Geometry: final body of the model. Coordinates: model frame, mm. A direction names the side the tool comes from. Give positions to 0.01 mm unless a question says otherwise; leave off trailing zeros. Loops run counter-clockwise (first coordinate to the right, second up) from the corner with the lowest first, then second, coordinate; pieces in that order, holes last. Notation, with made-up numbers: (67, 73.5) -> (95, 73.5) arc R15 ccw to (95, 90.5) -> close; hole circle Ø1 at (84, -8). An arc over 180 degrees is marked (long way). Answer in a Markdown table with one row per item. Add a question column.
1) Section query A-A (y = 148). Return the cut outline in (x, z), plus the area to 3 significant figures.
2) Line query: line 1 (Y direction, x = 0, z = 0.55); line 2 (Y direction, x = 48.5, z = 1.8); line 3 (Y direction, x = -71, z = 1.4). Output: solid intervals per line, ascending. Write a range as from..to.
3) Access query for faces 5 (the flat face through (73.772, 0.454, 0.986)), 6 (the flat face through (-61.02, 229.27, 0.99)), 7 (the flat face through (61.023, -14.957, 0.986)). Directions: +Z, -Z, +X, -X, +Y, -Y. A direction counts if a zero-diameter tool reaches every point of the face in a straight line with its end or side. Return the directions, or none.
4) Section query B-B (z = 1.3). Give the number of separate pieces and of enclosed holes in the cut face, plus the area to 3 significant figures.
5) First-contact query: P1, Ø1.3, axis at x = 74.81, y = 99.66, coming from the -Z side; P2, Ø1, axis at x = 80, z = 0.5, coming from the -Y side. Flat tips, straight axial feed; report the tip coordinate or a pass-through.
6) Draft query along Y for faces 1 (the flat face through (71.318, -10.358, 0.986)), 2 (the cylindrical face through (-58.96, 16.71, 0.99)), 3 (the cylindrical face through (59.714, 124.35, 0.986)), 4 (the flat face through (1, 109, 0)). Return one class per face: +Y half, -Y half, draft (parallel to the pull), parting line (faces both ways), or undercut.
7) Section query C-C (x = -30). Return the cut outline in (y, z), plus the area to 3 significant figures.
```python
from build123d import *

# Parameters (mm, degrees)
EXTRUDE_1_DEPTH     = 2
SKETCH_2_R          = 0.8
SKETCH_2_R_2        = 2
CUT_EXTRUDE_1_DEPTH = 10
SKETCH_3_R          = 1.5
SKETCH_3_R_2        = 1
CUT_EXTRUDE_2_DEPTH = 249.131112982
SKETCH_4_R          = 2
CUT_EXTRUDE_3_DEPTH = 10


with BuildPart() as part:
    # 草图1 → 凸台-拉伸1 (new body)
    with BuildSketch(Plane.XY):
        with BuildLine():
            Line((-52.894125512, 33.242924291), (-52.894125512, 73.242924291))
            ThreePointArc((-52.894125512, 73.242924291), (-59.898712726, 90.153493742), (-76.809282177, 97.158080957))
            Line((-76.809282177, 97.158080957), (-86.809282177, 97.158080957))
            Line((-86.809282177, 97.158080957), (-86.809282177, 117.158080957))
            Line((-86.809282177, 117.158080957), (-76.809282177, 117.158080957))
            ThreePointArc((-76.809282177, 117.158080957), (-59.898712726, 124.162668171), (-52.894125512, 141.073237622))
            Line((-52.894125512, 141.073237622), (-52.894125512, 181.073237622))
            ThreePointArc((-52.894125512, 181.073237622), (-58.833242973, 197.390828739), (-69.995132678, 210.693050895))
            Line((-69.995132678, 210.693050895), (-77.655577109, 217.120926992))
            Line((-77.655577109, 217.120926992), (-64.799824916, 232.441815854))
            Line((-64.799824916, 232.441815854), (-57.139380484, 226.013939757))
            ThreePointArc((-57.139380484, 226.013939757), (-42.101007166, 217.331530874), (-25, 214.316161913))
            Line((-25, 214.316161913), (25, 214.316161913))
            ThreePointArc((25, 214.316161913), (42.101007166, 217.331530874), (57.139380484, 226.013939757))
            Line((57.139380484, 226.013939757), (64.799824916, 232.441815854))
            Line((64.799824916, 232.441815854), (77.655577109, 217.120926992))
            Line((77.655577109, 217.120926992), (69.995132678, 210.693050895))
            ThreePointArc((69.995132678, 210.693050895), (58.833242973, 197.390828739), (52.894125512, 181.073237622))
            Line((52.894125512, 181.073237622), (52.894125512, 141.073237622))
            ThreePointArc((52.894125512, 141.073237622), (59.898712726, 124.162668171), (76.809282177, 117.158080957))
            Line((76.809282177, 117.158080957), (86.809282177, 117.158080957))
            Line((86.809282177, 117.158080957), (86.809282177, 97.158080957))
            Line((86.809282177, 97.158080957), (76.809282177, 97.158080957))
            ThreePointArc((76.809282177, 97.158080957), (59.898712726, 90.153493742), (52.894125512, 73.242924291))
            Line((52.894125512, 73.242924291), (52.894125512, 33.242924291))
            ThreePointArc((52.894125512, 33.242924291), (58.833242973, 16.925333174), (69.995132678, 3.623111018))
            Line((69.995132678, 3.623111018), (77.655577109, -2.804765079))
            Line((77.655577109, -2.804765079), (64.799824916, -18.125653941))
            Line((64.799824916, -18.125653941), (57.139380484, -11.697777844))
            ThreePointArc((57.139380484, -11.697777844), (42.101007166, -3.015368961), (25, 0))
            Line((25, 0), (-25, 0))
            ThreePointArc((-25, 0), (-42.101007166, -3.015368961), (-57.139380484, -11.697777844))
            Line((-57.139380484, -11.697777844), (-64.799824916, -18.125653941))
            Line((-64.799824916, -18.125653941), (-77.655577109, -2.804765079))
            Line((-77.655577109, -2.804765079), (-69.995132678, 3.623111018))
            ThreePointArc((-69.995132678, 3.623111018), (-58.833242973, 16.925333174), (-52.894125512, 33.242924291))
        make_face()
    extrude(amount=EXTRUDE_1_DEPTH)

    # 草图2 → 切除-拉伸1 (cut)
    with BuildSketch(Plane.XY.offset(2)):
        with Locations((-62.035167695, 217.067920107)):
            Circle(SKETCH_2_R)
        with Locations((-71.896992065, 216.205122273)):
            Circle(SKETCH_2_R)
        with Locations((-62.897965529, 226.929744476)):
            Circle(SKETCH_2_R)
        with Locations((-81.809282177, 100.158080957)):
            Circle(SKETCH_2_R)
        with Locations((-74.809282177, 107.158080957)):
            Circle(SKETCH_2_R)
        with Locations((-81.809282177, 114.158080957)):
            Circle(SKETCH_2_R)
        with Locations((81.809282177, 114.158080957)):
            Circle(SKETCH_2_R)
        with Locations((74.809282177, 107.158080957)):
            Circle(SKETCH_2_R)
        with Locations((81.809282177, 100.158080957)):
            Circle(SKETCH_2_R)
        with Locations((71.896992065, 216.205122273)):
            Circle(SKETCH_2_R)
        with Locations((62.035167695, 217.067920107)):
            Circle(SKETCH_2_R)
        with Locations((62.897965529, 226.929744476)):
            Circle(SKETCH_2_R)
        with Locations((71.896992065, -1.888960359)):
            Circle(SKETCH_2_R)
        with Locations((62.035167695, -2.751758193)):
            Circle(SKETCH_2_R)
        with Locations((62.897965529, -12.613582563)):
            Circle(SKETCH_2_R)
        with Locations((-71.896992065, -1.888960359)):
            Circle(SKETCH_2_R)
        with Locations((-62.035167695, -2.751758193)):
            Circle(SKETCH_2_R)
        with Locations((-62.897965529, -12.613582563)):
            Circle(SKETCH_2_R)
        with Locations((-47.894125512, 63.242924291)):
            Circle(SKETCH_2_R_2)
        with Locations((-47.894125512, 43.242924291)):
            Circle(SKETCH_2_R_2)
        with Locations((47.894125512, 43.242924291)):
            Circle(SKETCH_2_R_2)
        with Locations((47.894125512, 63.242924291)):
            Circle(SKETCH_2_R_2)
        with Locations((-10, 5)):
            Circle(SKETCH_2_R_2)
        with Locations((10, 5)):
            Circle(SKETCH_2_R_2)
        with Locations((-74.809282177, 114.658080957)):
            Circle(SKETCH_2_R)
        with Locations((-74.809282177, 99.658080957)):
            Circle(SKETCH_2_R)
        with Locations((74.809282177, 114.658080957)):
            Circle(SKETCH_2_R)
        with Locations((74.809282177, 99.658080957)):
            Circle(SKETCH_2_R)
        with Locations((66.856074768, 2.99357513)):
            Circle(SKETCH_2_R)
        with Locations((57.214260622, -8.497091517)):
            Circle(SKETCH_2_R)
        with Locations((-57.214260622, -8.497091517)):
            Circle(SKETCH_2_R)
        with Locations((-66.856074768, 2.99357513)):
            Circle(SKETCH_2_R)
        with Locations((-57.214260622, 222.81325343)):
            Circle(SKETCH_2_R)
        with Locations((-66.856074768, 211.322586783)):
            Circle(SKETCH_2_R)
        with Locations((66.856074768, 211.322586783)):
            Circle(SKETCH_2_R)
        with Locations((57.214260622, 222.81325343)):
            Circle(SKETCH_2_R)
    extrude(amount=-CUT_EXTRUDE_1_DEPTH, mode=Mode.SUBTRACT)

    # 草图3 → 切除-拉伸2 (cut, through all)
    with BuildSketch(Plane.XY.offset(2)):
        with Locations((0, 53.242924291)):
            Circle(SKETCH_3_R)
        with Locations((0, 60.242924291)):
            Circle(SKETCH_3_R_2)
        with Locations((7, 53.242924291)):
            Circle(SKETCH_3_R_2)
        with Locations((0, 46.242924291)):
            Circle(SKETCH_3_R_2)
        with Locations((-7, 53.242924291)):
            Circle(SKETCH_3_R_2)
    extrude(amount=-CUT_EXTRUDE_2_DEPTH, mode=Mode.SUBTRACT)

    # 草图4 → 切除-拉伸3 (cut)
    with BuildSketch(Plane.XY.offset(2)):
        with Locations((4, 161.073237622)):
            Circle(SKETCH_4_R)
        with Locations((-4, 161.073237622)):
            Circle(SKETCH_4_R)
    extrude(amount=-CUT_EXTRUDE_3_DEPTH, mode=Mode.SUBTRACT)


solid = part.part
```
Evaluation:
| question | item | result |
|---|---|---|
| 1 | outline | (-52.89, 0) -> (52.89, 0) -> (52.89, 2) -> (-52.89, 2) -> close |
| 1 | area | 212 mm² |
| 2 | line 1 | 0..45.24, 47.24..51.74, 54.74..59.24, 61.24..214.32 |
| 2 | line 2 | -5.87..41.34, 45.15..61.34, 65.15..220.18 |
| 2 | line 3 | -10.74..2.78, 96.44..117.87, 211.54..225.05 |
| 3 | face 5 | +Z, -Z, +X |
| 3 | face 6 | +Z, -Z, +Y |
| 3 | face 7 | +Z, -Z, -Y |
| 4 | separate pieces | 1 |
| 4 | enclosed holes | 43 |
| 4 | area | 26,800 mm² |
| 5 | P1 | through |
| 5 | P2 | y = 97.16 |
| 6 | face 1 | -Y half |
| 6 | face 2 | undercut |
| 6 | face 3 | undercut |
| 6 | face 4 | draft |
| 7 | outline | (-0.25, 0) -> (214.57, 0) -> (214.57, 2) -> (-0.25, 2) -> close |
| 7 | area | 430 mm² |
